Check sheet for the drawn part. Datum: minimum x, y, z corner. Units: mm. Give positions to 0.01 mm unless a question says otherwise; leave off trailing zeros. Order: outer loops, then holes, each group sorted by start corner. A loop starts at its lowest first (then second) coordinate and runs counter-clockwise, first axis right, second up.
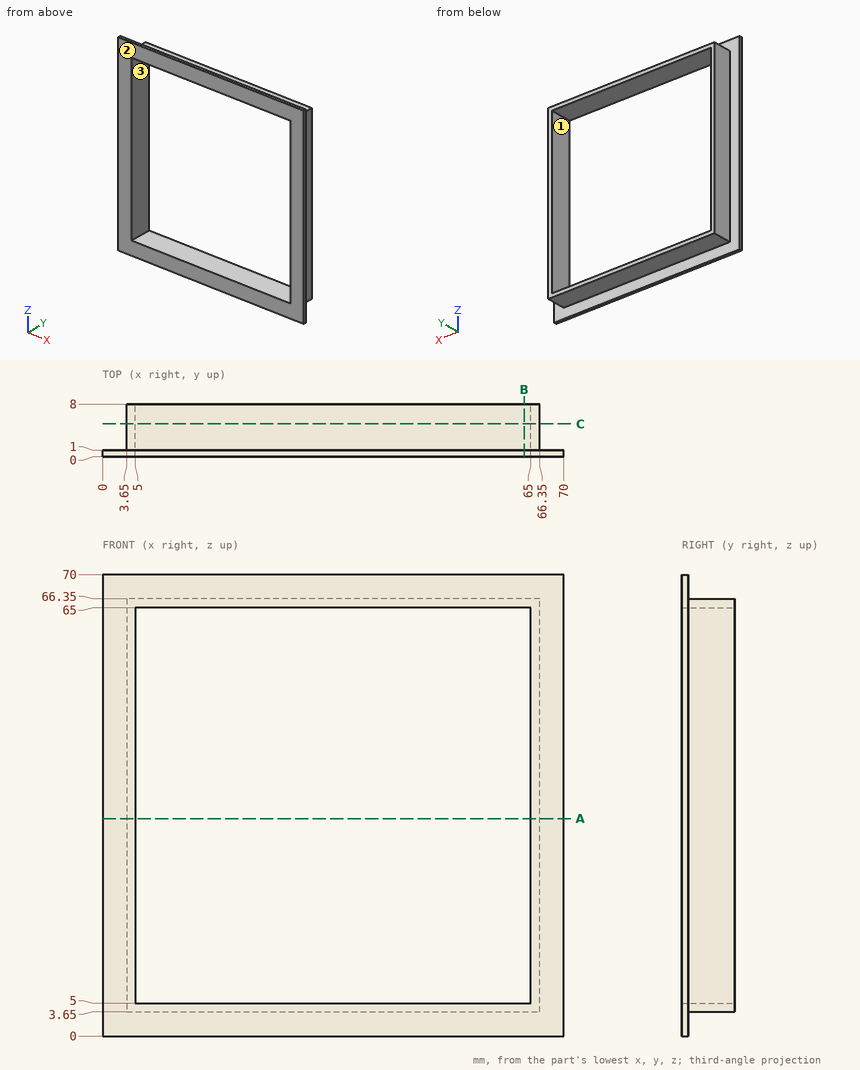
Q1. Draft check along Z on the marked faces 1, 2 and 3. Enter one of: pulls with the +Z half, pulls with the -Z half, needs draft (parallel to the pull), parting line crosses it, or undercut.
Q2. Material ranges on line 1 (Z direction, x = 40.5, y = 4.5), recorded low to high.
Q3. Go/stop test with flat-tipped pins: P1, Ø1.5, axis at y = 4, z = 12, coming from the +X side; P2, Ø2, axis at y = 4, z = 36, coming from the -X side; P3, Ø2, axis at x = 37.5, y = 6, coming from the -Z side. Record where each tip stops, or that it passes through.
Q4. Sectioned sample at B-B, the plane x = 64. Record the cut outline in (y, z), plus the area to 3 significant figures.
Q5. Sectioned sample at A-A, the plane z = 33. Record the cut outline in (x, y).
Q6. Sectioned sample at C-C, the plane y = 5. Record the cut outline in (x, z).
Filled in:
1. face 1: undercut
1. face 2: needs draft
1. face 3: undercut
2. line 1: z = 3.65 to 5, 65 to 66.35
3. P1: stops at x = 66.35
3. P2: stops at x = 3.65
3. P3: stops at z = 3.65
4. outline: (0, 0) - (1, 0) - (1, 3.65) - (8, 3.65) - (8, 5) - (0, 5) - close; (0, 65) - (8, 65) - (8, 66.35) - (1, 66.35) - (1, 70) - (0, 70) - close
4. area: 28.9 mm2
5. outline: (0, 0) - (5, 0) - (5, 8) - (3.65, 8) - (3.65, 1) - (0, 1) - close; (65, 0) - (70, 0) - (70, 1) - (66.35, 1) - (66.35, 8) - (65, 8) - close
6. outline: (3.65, 3.65) - (66.35, 3.65) - (66.35, 66.35) - (3.65, 66.35) - close; hole (5, 5) - (65, 5) - (65, 65) - (5, 65) - close
